Autodesk Fusion 360 part; units mm, degrees
sketch "Sketch1" plane through (0, 0, 0) normal (0, 0, 1) x (1, 0, 0) in component "exercise 2"
  circle A0 centre (0, 0) radius 30
  line L0 (0, 0) -> (129, 0) construction
  circle A1 centre (129, 0) radius 20
  line L1 (0, 0) -> (0, 74.6683) construction
  line L2 (129, 0) -> (129, 70.5762) construction
  line L3 (-20, 0) -> (-10, -17.3205)
  line L4 (-10, -17.3205) -> (10, -17.3205)
  line L5 (10, -17.3205) -> (20, 0)
  line L6 (20, 0) -> (10, 17.3205)
  line L7 (10, 17.3205) -> (-10, 17.3205)
  line L8 (-10, 17.3205) -> (-20, 0)
  line L9 (129, 15) -> (114.7342, 4.6353)
  line L10 (114.7342, 4.6353) -> (120.1832, -12.1353)
  line L11 (120.1832, -12.1353) -> (137.8168, -12.1353)
  line L12 (137.8168, -12.1353) -> (143.2658, 4.6353)
  line L13 (143.2658, 4.6353) -> (129, 15)
  line L14 (30, 0) -> (31.5826, 0)
  line L15 (28.2843, 10) -> (111.6795, 10)
  line L16 (28.2843, -10) -> (111.6795, -10)
  line L17 (50, 10) -> (50, -10) construction
  line L18 (50, 0) -> (52, 0)
  line L19 (99.5, -5) -> (39.5, -5)
  line L20 (39.5, 5) -> (99.5, 5)
  line L21 (99.5, -5) -> (39.5, 5) construction
  line L22 (39.5, -5) -> (99.5, 5) construction
  arc A2 (41.1216, 4.7297) -> (41.1216, -4.7297) centre (39.5, 0) ccw
  arc A3 (97.8784, -4.7297) -> (97.8784, 4.7297) centre (99.5, 0) ccw
  point P0 (129, 0)
  point P1 (69.5, 0)
  dimension "d1" = 60
  dimension "d2" = 40
  dimension "d3" = 129
  dimension "d4" = 20
  dimension "d5" = 15
  dimension "d6" = 20
  dimension "d9" = 60
extrude "Extrude1" add sketch "Sketch1" along normal mid plane 20 contours A0 | A1 makes body 1 at (18.836, -10.4559, 10) makes body 2 at (148.9006, -1.9914, -3.3333) in component "exercise 2"
extrude "Extrude2" add sketch "Sketch1" along normal mid plane 12 contours A0 A1 L15 L16 bodies 1 2 in component "exercise 2"
extrude "Extrude3" add sketch "Sketch1" along normal mid plane 6 contours L19 L20 A2 A3 bodies 1 in component "exercise 2"
component "exercise 2" placed x (1, 0, 0) y (0, 1, 0) z (0, 0, 1) at (0, 0, 0)
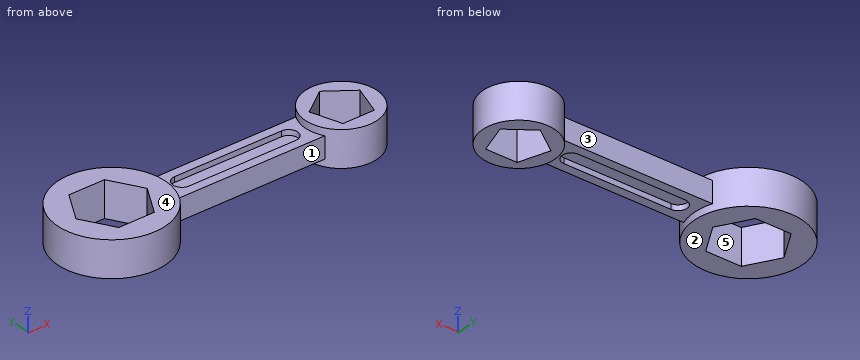
Verification items for the finished model (mm, model axes). Face numbers are marked on the shaded views. A direction names the side the tool comes from. Give positions to 0.01 mm unless a question says otherwise; leave off trailing zeros. Order: outer loops, then holes, each group sorted by start corner. A loop starts at its lowest first (then second) coordinate and runs counter-clockwise, first axis right, second up. Notation, with made-up numbers: (81.25, 51) -> (130.25, 51) arc R19 cw to (130.25, 70) -> close; hole circle Ø9 at (-25, -31.5). An arc over 180 degrees is marked (long way). One line per item, written item: value.
(1) Gauge pin test, flat ends, axial feed: pin 1 (3 mm diameter, centred on x = 86, y = 2.5, fed in from -Z); pin 2 (5 mm diameter, centred on x = 48, z = -5, fed in from -Y); pin 3 (3.5 mm diameter, centred on x = 65, z = 5, fed in from +Y); pin 4 (10 mm diameter, centred on x = 117, y = 18, fed in from +Z). Record the tip position at first contact, or that the pin passes through.
Final values:
pin 1: z = -3
pin 2: y = -10
pin 3: y = 10
pin 4: z = 10
(2) Sectioned sample at C-C on y = 2. Record the cut outline in (x, z), then the cut area to 3 significant figures.
Final values:
outline: (-29.93, -10) -> (-18.85, -10) -> (-18.85, 10) -> (-29.93, 10) -> close; (18.85, -10) -> (29.93, -10) -> (29.93, -6) -> (34.92, -6) -> (34.92, -3) -> (104.08, -3) -> (104.08, -6) -> (109.1, -6) -> (109.1, -10) -> (115.59, -10) -> (115.59, 10) -> (109.1, 10) -> (109.1, 6) -> (104.08, 6) -> (104.08, 3) -> (34.92, 3) -> (34.92, 6) -> (29.93, 6) -> (29.93, 10) -> (18.85, 10) -> close; (142.41, -10) -> (148.9, -10) -> (148.9, 10) -> (142.41, 10) -> close
area: 1,240 mm^2
(3) Scan lines: line 1 along Y through (x, z) = (44, 3.5); line 2 along X through (y, z) = (9, 5.5); line 3 along X through (y, z) = (15.5, 3.5). Record each from-to range of solid material in increasing order. Write a range as [from, to].
Final values:
line 1: [-10, -5], [5, 10]
line 2: [-28.62, -14.8], [14.8, 120.74], [137.26, 146.86]
line 3: [-25.69, -11.05], [11.05, 25.69], [116.36, 141.64]
(4) Sectioned sample at D-D on y = -15. Record the cut outline in (x, z).
Final values:
outline: (-25.98, -10) -> (-11.34, -10) -> (-11.34, 10) -> (-25.98, 10) -> close; (11.34, -10) -> (25.98, -10) -> (25.98, 10) -> (11.34, 10) -> close; (115.77, -10) -> (142.23, -10) -> (142.23, 10) -> (115.77, 10) -> close
(5) Tool access check on the marked faces 3, 4 and 5. Record the directions out of +Z, -Z, +X, -X, +Y, -Y that give a thin tool (end or side, any length) a straight path to the whole face; none if there is none.
Final values:
face 3: +Z, -Z, +Y
face 4: +Z, +X, -X, +Y, -Y
face 5: +Z, -Z
(6) Draft check along X on the marked faces 1 and 2. Enter one of: pulls with the +X half, pulls with the -X half, needs draft (parallel to the pull), parting line crosses it, or undercut.
Final values:
face 1: undercut
face 2: needs draft
(7) Sectioned sample at A-A on x = 0. Record the cut outline in (y, z), then the cut area to 3 significant figures.
Final values:
outline: (-30, -10) -> (-17.32, -10) -> (-17.32, 10) -> (-30, 10) -> close; (17.32, -10) -> (30, -10) -> (30, 10) -> (17.32, 10) -> close
area: 507 mm^2
(8) Sectioned sample at B-B on z = -1. Record the cut outline in (x, y).
Final values:
outline: (28.28, -10) -> (111.68, -10) arc R20 ccw (long way) to (111.68, 10) -> (28.28, 10) arc R30 ccw (long way) to start; hole (-20, 0) -> (-10, -17.32) -> (10, -17.32) -> (20, 0) -> (10, 17.32) -> (-10, 17.32) -> close; hole (114.73, 4.64) -> (120.18, -12.14) -> (137.82, -12.14) -> (143.27, 4.64) -> (129, 15) -> close
